Build history of the part. All positions in model axes, mm. A direction names the side the tool comes from. Give positions to 0.01 mm unless a question says otherwise; leave off trailing zeros. Loops run counter-clockwise (first coordinate to the right, second up) from the corner with the lowest first, then second, coordinate; pieces in that order, holes last. Notation, with made-up numbers: (68.5, 52) -> (89.5, 52) arc R31 cw to (89.5, 88) -> close; hole circle Ø10 at (-3.5, 28). An arc over 180 degrees is marked (long way). One line per question, with ' | ' between items. Start each with the question number.
(1) Slice it at B-B, the plane x = -32.75. Write the cut outline in (y, z), then the cut area to 3 significant figures.
(2) Slice it at D-D, the plane x = -35.5. Write the cut outline in (y, z), then the cut area to 3 significant figures.
(3) Slice it at C-C, the plane z = 19.75. Write the cut outline in (x, y).
(4) Drill centre line: L1, parallel to Y at x = -43.75, z = 16.3. Where is it in solid material? Low to high. Write a range as from..to.
(5) 3-axis set-ups, long thin cutter, end or side, ignore diameter. For faces 1 (the face through (-32.545, 12.493, 18.926)), 2 (the face through (-38, 0, 18)): which of +Z, -Z, +X, -X, +Y, -Y reach the whole face in a straight line?
(6) Slice it at A-A, the plane z = 18.45. Write the cut outline in (x, y), then the cut area to 3 significant figures.
```python
from build123d import *

# Parameters (mm, degrees)
SKETCH_1_W          = 13.3
SKETCH_1_H          = 5
EXTRUDE_1_DEPTH     = 12
SKETCH_2_R          = 1
EXTRUDE_2_DEPTH     = 1
SKETCH_3_W          = 2.738665781
SKETCH_3_H          = 0.337471602
CUT_EXTRUDE_1_DEPTH = 0.4


with BuildPart() as part:
    # Эскиз1 → Бобышка-Вытянуть1 (new body)
    with BuildSketch(Plane(origin=(0, 0, 0), x_dir=(1, 0, 0), z_dir=(0, 1, 0))):
        with Locations((-38.349307958, -18.52646235)):
            Rectangle(SKETCH_1_W, SKETCH_1_H)
    extrude(amount=EXTRUDE_1_DEPTH)

    # Эскиз2 → Бобышка-Вытянуть2 (add)
    with BuildSketch(Plane(origin=(0, 12, 0), x_dir=(1, 0, 0), z_dir=(0, 1, 0))):
        with Locations((-33.499307958, -19.22646235)):
            Circle(SKETCH_2_R)
    extrude(amount=EXTRUDE_2_DEPTH)

    # Эскиз3 → Вырез-Вытянуть1 (cut)
    with BuildSketch(Plane(origin=(0, 13, 0), x_dir=(1, 0, 0), z_dir=(0, 1, 0))):
        with Locations((-33.499307958, -19.22646235)):
            Rectangle(SKETCH_3_W, SKETCH_3_H)
    extrude(amount=-CUT_EXTRUDE_1_DEPTH, mode=Mode.SUBTRACT)


solid = part.part
```
Final values:
1) outline: (0, 16.03) -> (12, 16.03) -> (12, 18.56) -> (13, 18.56) -> (13, 19.06) -> (12.6, 19.06) -> (12.6, 19.4) -> (13, 19.4) -> (13, 19.89) -> (12, 19.89) -> (12, 21.03) -> (0, 21.03) -> close | area: 61.2 mm2
2) outline: (0, 16.03) -> (12, 16.03) -> (12, 21.03) -> (0, 21.03) -> close | area: 60.0 mm2
3) outline: (-45, 0) -> (-31.7, 0) -> (-31.7, 12) -> (-32.65, 12) -> (-32.65, 13) -> (-34.35, 13) -> (-34.35, 12) -> (-45, 12) -> close
4) L1: 0..12
5) face 1: +Y | face 2: +Z, -Z, +X, -X, -Y
6) outline: (-45, 0) -> (-31.7, 0) -> (-31.7, 12) -> (-32.87, 12) -> (-32.87, 13) -> (-34.13, 13) -> (-34.13, 12) -> (-45, 12) -> close | area: 161 mm2
